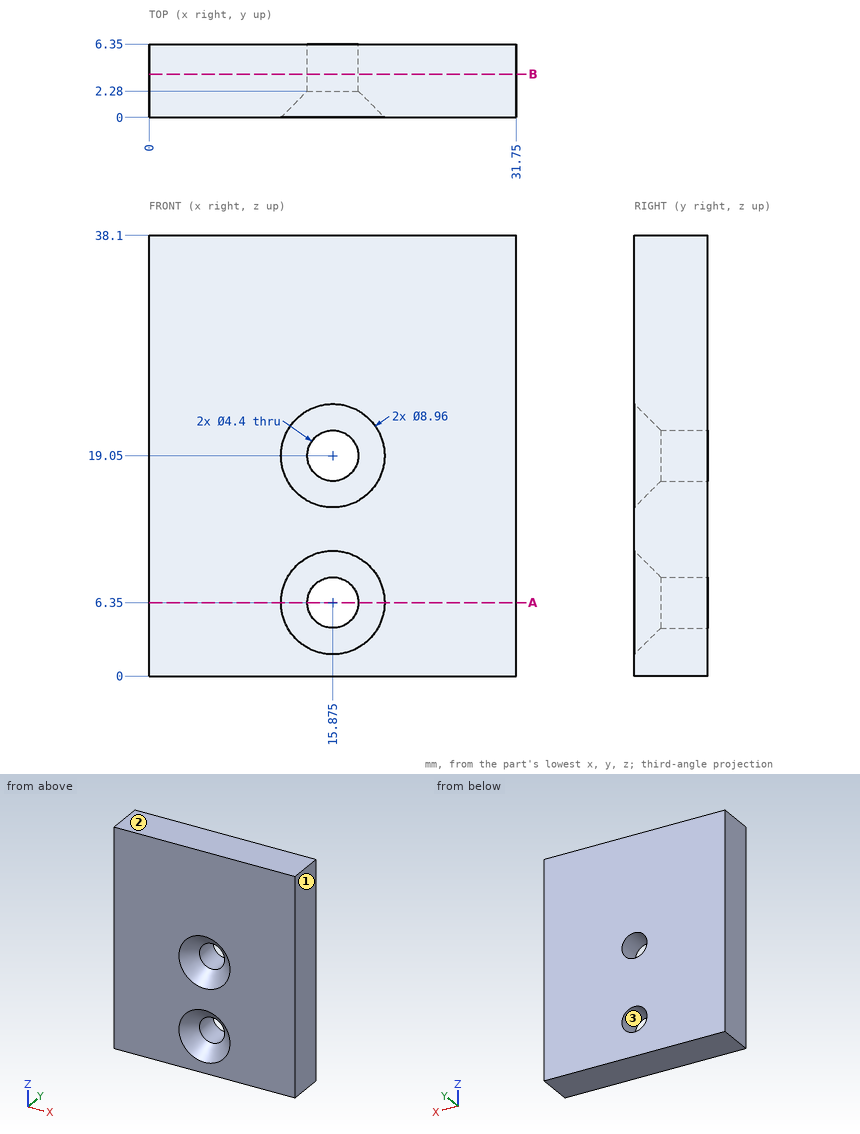
Job drawing, mm, ordinate dimensions from the low corner. One solid piece. Give positions to 0.01 mm unless a question says otherwise; leave off trailing zeros. Loops run counter-clockwise (first coordinate to the right, second up) from the corner with the lowest first, then second, coordinate; pieces in that order, holes last. Notation, with made-up numbers: (4.25, -11) -> (54.25, -11) arc R15 ccw to (54.25, -7) -> close; hole circle Ø10 at (45, 4.5). An arc over 180 degrees is marked (long way). Use a Markdown table: item, result. Add a question column.
(1) Drop a flat-ended pin along its axis: pin 1 Ø7 at (x, z) = (15.875, 19.05) entering from -Y. Give the stop position or say it passes through.
(2) Slice it at A-A on z = 6.35. List the corners of the cut face in (x, y) (3 decimals).
(3) Wall check: line 1 along X through (y, z) = (4, 19.05) (3 decimals); line 2 along Z through (x, y) = (15, 1.5); line 3 along X through (y, z) = (0.5, 6). Give the ranges that are in metal, low to high.
(4) Slice it at B-B on y = 3.75. List the corners of the cut face in (x, z) (3 decimals), and give its area (3 significant figures).
(5) Mould opens along X. For the marked faces 1, 2 and 3 say: +X half, -X half, draft (parallel to the pull), parting line (faces both ways), or undercut.
Filled sheet:
| question | item | result |
|---|---|---|
| 1 | pin 1 | y = 0.98 |
| 2 | outline | (0, 0) -> (11.395, 0) -> (13.675, 2.28) -> (13.675, 6.35) -> (0, 6.35) -> close; (18.075, 2.28) -> (20.355, 0) -> (31.75, 0) -> (31.75, 6.35) -> (18.075, 6.35) -> close |
| 3 | line 1 | 0 to 13.675, 18.075 to 31.75 |
| 3 | line 2 | 0 to 3.5, 9.2 to 16.2, 21.9 to 38.1 |
| 3 | line 3 | 0 to 11.91, 19.84 to 31.75 |
| 4 | outline | (0, 0) -> (31.75, 0) -> (31.75, 38.1) -> (0, 38.1) -> close; hole circle Ø4.4 at (15.875, 6.35); hole circle Ø4.4 at (15.875, 19.05) |
| 4 | area | 1,180 mm2 |
| 5 | face 1 | +X half |
| 5 | face 2 | draft |
| 5 | face 3 | undercut |
